Geometry check sheet. Reference: the model listing, model coordinates, mm. A direction names the side the tool comes from. Coordinates: 2 decimals unless noted, no trailing zeros. Order: outer loops, then holes, each group sorted by start corner. A loop starts at its lowest first (then second) coordinate and runs counter-clockwise, first axis right, second up. Notation, with made-up numbers: (78.25, 10.5) - (100.25, 10.5) arc R18 ccw to (100.25, 43.5) - close; hole circle Ø1 at (41, 8). An arc over 180 degrees is marked (long way). Use CSV: the item, a comma, the result in double quotes. Start each with the question number.
1) Draft check along Z on faces 4 (the flat face through (1, 0.5, 21)), 5 (the flat face through (6, 1, 22)), 6 (the flat face through (2.373, -0.5, 16.1)), 7 (the flat face through (1, 0.5, 2)). Enter one of: released by +Z, released by -Z, zero draft, split by the parting line, or undercut.
2) Sectioned sample at A-A, the plane y = -0.3. Record the cut outline in (x, z).
3) Sectioned sample at C-C, the plane x = 4. Record the cut outline in (y, z), and give its area (3 significant figures).
4) Depth check by flat-ended pin: P1, Ø2.5, axis at x = 4, z = 21, coming from the -Y side; P2, Ø0.8, axis at y = -0.5, z = 9, coming from the -X side; P3, Ø0.5, axis at y = -0.5, z = 5, coming from the +X side; P4, Ø1.1, axis at y = -0.5, z = 16.5, coming from the +X side. Enter the tip coordinate at first touch or a pass-through.
5) Thickness scan on probe 1 along X at (y, z) = (0.4, 21); probe 2 along Z at (x, y) = (4, 0.25); probe 3 along Z at (x, y) = (2.75, -0.3). Record the ranges inside material, lowest first. Write a range as [from, to].
6) Sectioned sample at D-D, the plane z = 11.25. Record the cut outline in (x, y), and give its area (3 significant figures).
7) Sectioned sample at B-B, the plane z = 15.75. Record the cut outline in (x, y).
8) Tool access check on faces 1 (the flat face through (4, -0.5, 8)), 2 (the flat face through (3.373, -0.5, 5.1)), 3 (the flat face through (6.906, -0.5, 5.1)). Record the directions out of +Z, -Z, +X, -X, +Y, -Y that give a thin tool (end or side, any length) a straight path to the whole face; none if there is none.
Autodesk Fusion 360 part; units mm, degrees
sketch "Boceto1" plane through (0, 0, 0) normal (0, 1, 0) x (1, 0, 0)
  line L0 (0, 0) -> (11, 0)
  line L1 (11, 0) -> (11, -22)
  line L2 (11, -22) -> (0, -22)
  line L3 (0, -22) -> (0, 0)
  dimension "d1" = 11
  dimension "d2" = 22
extrude "Extruir1" add sketch "Boceto1" along normal blind 2
sketch "Boceto2" plane through (0, 0, 0) normal (0, -1, 0) x (1, 0, 0)
  line L0 (11, 22) -> (0, 22)
  line L1 (0, 22) -> (0, 0)
  line L2 (0, 0) -> (11, 0)
  line L3 (11, 0) -> (11, 22)
  line L4 (8, 12) -> (10.1306, 12)
  line L5 (10.1306, 12) -> (10.1306, 8.6002)
  line L6 (10.1306, 8.6002) -> (8, 8.6002)
  line L7 (8, 8.6002) -> (8, 12)
  line L8 (2, 12) -> (6, 12)
  line L9 (6, 12) -> (6, 8)
  line L10 (6, 8) -> (2, 8)
  line L11 (2, 8) -> (2, 12)
extrude "Extruir2" add sketch "Boceto2" along normal blind 1 contours L4 L5 L6 L7 | L8 L9 L10 L11
sketch "Boceto3" plane through (0, 0, 0) normal (0, 1, 0) x (1, 0, 0)
  circle A0 centre (1.3364, -1.7459) radius 0.9984
  circle A1 centre (9.3364, -1.7459) radius 0.9984
  circle A2 centre (1, -21) radius 0.7455
  circle A3 centre (4, -21) radius 0.7455
extrude "Extruir3" cut sketch "Boceto3" along normal blind 0.5
sketch "Boceto4" plane through (0, 0, 0) normal (0, 1, 0) x (1, 0, 0)
  line L0 (3.3729, -5.8021) -> (6.9064, -5.8021)
  line L1 (6.9064, -5.8021) -> (6.9064, -4.4369)
  line L2 (6.9064, -4.4369) -> (3.3729, -4.4369)
  line L3 (3.3729, -4.4369) -> (3.3729, -5.8021)
  line L4 (2.3729, -16.8021) -> (5.9064, -16.8021)
  line L5 (5.9064, -15.4369) -> (2.3729, -15.4369)
  line L6 (2.3729, -15.4369) -> (2.3729, -16.8021)
  line L7 (5.9064, -16.8021) -> (5.9064, -15.4369)
extrude "Extruir5" add sketch "Boceto4" against normal blind 1
Evaluation:
1,face 4,"undercut"
1,face 5,"released by +Z"
1,face 6,"zero draft"
1,face 7,"undercut"
2,outline,"(2, 8) - (6, 8) - (6, 12) - (2, 12) - close; (2.37, 15.44) - (5.91, 15.44) - (5.91, 16.8) - (2.37, 16.8) - close; (3.37, 4.44) - (6.91, 4.44) - (6.91, 5.8) - (3.37, 5.8) - close; (8, 8.6) - (10.13, 8.6) - (10.13, 12) - (8, 12) - close"
3,outline,"(-1, 4.44) - (0, 4.44) - (0, 0) - (2, 0) - (2, 22) - (0, 22) - (0, 21.75) - (0.5, 21.75) - (0.5, 20.25) - (0, 20.25) - (0, 16.8) - (-1, 16.8) - (-1, 15.44) - (0, 15.44) - (0, 12) - (-1, 12) - (-1, 8) - (0, 8) - (0, 5.8) - (-1, 5.8) - close"
3,area,"50.0 mm²"
4,P1,"y = 0"
4,P2,"x = 2"
4,P3,"x = 6.91"
4,P4,"x = 11"
5,probe 1,"[0, 0.25], [1.75, 3.25], [4.75, 11]"
5,probe 2,"[0, 20.25], [21.75, 22]"
5,probe 3,"[8, 12], [15.44, 16.8]"
6,outline,"(0, 0) - (2, 0) - (2, -1) - (6, -1) - (6, 0) - (8, 0) - (8, -1) - (10.13, -1) - (10.13, 0) - (11, 0) - (11, 2) - (0, 2) - close"
6,area,"28.1 mm²"
7,outline,"(0, 0) - (2.37, 0) - (2.37, -1) - (5.91, -1) - (5.91, 0) - (11, 0) - (11, 2) - (0, 2) - close"
8,face 1,"+X, -X, -Y"
8,face 2,"-Z, -X, -Y"
8,face 3,"+Z, -Z, +X, -Y"
